For this review, take the finished solid that the model builds, in its own axes (mm). Coordinates: 2 decimals unless noted, no trailing zeros. Write each loop counter-clockwise with the first axis right and the second up, starting at its lowest first coordinate (ties: lowest second). Pieces come first, ordered by that corner, then holes. Notation, with made-up numbers: M 78.25,76 L 102.25,76 A16 cw 102.25,94 Z; hole C 17,-28.5 d10. An arc over 180 degrees is marked long. Return JSON: item names as keys, results as strings.
```python
from build123d import *

# Parameters (mm, degrees)
SKETCH1_W            = 158
SKETCH1_H            = 93
BOSS_EXTRUDE1_DEPTH  = 1.143
FILLET1_R            = 25
M4_CLEARANCE_HOLE1_D = 4.5
CHAMFER2_SIZE        = 2
CUT_EXTRUDE1_REACH   = 93.698
FILLET2_R            = 2


with BuildPart() as part:
    # Sketch1 → Boss-Extrude1 (new, symmetric)
    with BuildSketch(Plane.XY):
        Rectangle(SKETCH1_W, SKETCH1_H)
    extrude(amount=BOSS_EXTRUDE1_DEPTH, both=True)

    # Fillet1
    fillet1_edges = [part.edges().sort_by_distance(p)[0] for p in [
        (-79, 46.5, 0),
        (79, 46.5, 0),
        (79, -46.5, 0),
        (-79, -46.5, 0),
    ]]
    fillet(fillet1_edges, radius=FILLET1_R)

    # M4 Clearance Hole1 (through all)
    with Locations(Plane.XY.offset(1.143)):
        with Locations((72.5, 12.5), (0, 40), (0, -40), (-36.25, -40), (-36.25, 40), (36.25, 40), (36.25, -40), (-64.814123615, 35.759516477), (-64.814123615, -35.759516477), (64.814123615, -35.759516477), (64.814123615, 35.759516477), (-72.5, 12.5), (-72.5, -12.5), (72.5, -12.5)):
            Hole(M4_CLEARANCE_HOLE1_D / 2)

    # Chamfer2
    chamfer2_edges = [part.edges().sort_by_distance(p)[0] for p in [
        (-79, 0, 1.143),
        (0, 46.5, 1.143),
        (0, -46.5, 1.143),
        (79, 0, 1.143),
        (71.67766953, 39.17766953, 1.143),
        (-71.67766953, -39.17766953, 1.143),
        (71.67766953, -39.17766953, 1.143),
        (-71.67766953, 39.17766953, 1.143),
    ]]
    chamfer(chamfer2_edges, length=CHAMFER2_SIZE)

    # Sketch7 → Cut-Extrude1 (cut, up to next)
    with BuildSketch(Plane.XY.offset(1.143), mode=Mode.PRIVATE) as cut_extrude1_sk1:
        with BuildLine():
            Line((-33, 19.211525688), (-33, 8.788474312))
            ThreePointArc((-33, 8.788474312), (-52.4, 14), (-33, 19.211525688))
        make_face()
    cut_extrude1_tool1 = extrude(cut_extrude1_sk1.sketch, amount=-CUT_EXTRUDE1_REACH, mode=Mode.PRIVATE) & part.part
    # Sketch7 → Cut-Extrude1 (cut, up to next)
    with BuildSketch(Plane.XY.offset(1.143), mode=Mode.PRIVATE) as cut_extrude1_sk2:
        with BuildLine():
            Line((-29.633180425, -5.65), (-22.366819575, -5.65))
            ThreePointArc((-22.366819575, -5.65), (-26, -22.15), (-29.633180425, -5.65))
        make_face()
    cut_extrude1_tool2 = extrude(cut_extrude1_sk2.sketch, amount=-CUT_EXTRUDE1_REACH, mode=Mode.PRIVATE) & part.part
    # Sketch7 → Cut-Extrude1 (cut, up to next)
    with BuildSketch(Plane.XY.offset(1.143), mode=Mode.PRIVATE) as cut_extrude1_sk3:
        with BuildLine():
            Line((-1, 19.211525688), (-1, 8.788474312))
            ThreePointArc((-1, 8.788474312), (-20.4, 14), (-1, 19.211525688))
        make_face()
    cut_extrude1_tool3 = extrude(cut_extrude1_sk3.sketch, amount=-CUT_EXTRUDE1_REACH, mode=Mode.PRIVATE) & part.part
    # Sketch7 → Cut-Extrude1 (cut, up to next)
    with BuildSketch(Plane.XY.offset(1.143), mode=Mode.PRIVATE) as cut_extrude1_sk4:
        with BuildLine():
            Line((31.197, 15.790698663), (31.197, 4.209301337))
            ThreePointArc((31.197, 4.209301337), (42.5, -2.7), (53.803, 4.209301337))
            Line((53.803, 4.209301337), (53.803, 15.790698663))
            ThreePointArc((53.803, 15.790698663), (42.5, 22.7), (31.197, 15.790698663))
        make_face()
    cut_extrude1_tool4 = extrude(cut_extrude1_sk4.sketch, amount=-CUT_EXTRUDE1_REACH, mode=Mode.PRIVATE) & part.part
    # Sketch7 → Cut-Extrude1 (cut, up to next)
    with BuildSketch(Plane.XY.offset(1.143), mode=Mode.PRIVATE) as cut_extrude1_sk5:
        with BuildLine():
            Line((9.49200639, -2.65), (19.50799361, -2.65))
            ThreePointArc((19.50799361, -2.65), (14.5, -23.55), (9.49200639, -2.65))
        make_face()
    cut_extrude1_tool5 = extrude(cut_extrude1_sk5.sketch, amount=-CUT_EXTRUDE1_REACH, mode=Mode.PRIVATE) & part.part
    add(cut_extrude1_tool1.solids().sort_by_distance((-42.286012, 14, 1.143))[0], mode=Mode.SUBTRACT)
    add(cut_extrude1_tool2.solids().sort_by_distance((-26, -13.638318, 1.143))[0], mode=Mode.SUBTRACT)
    add(cut_extrude1_tool3.solids().sort_by_distance((-10.286012, 14, 1.143))[0], mode=Mode.SUBTRACT)
    add(cut_extrude1_tool4.solids().sort_by_distance((42.5, 10, 1.143))[0], mode=Mode.SUBTRACT)
    add(cut_extrude1_tool5.solids().sort_by_distance((14.5, -12.722997, 1.143))[0], mode=Mode.SUBTRACT)

    # Fillet2
    fillet2_edges = [part.edges().sort_by_distance(p)[0] for p in [
        (31.197, 15.790698663, 0),
        (53.803, 15.790698663, 0),
        (53.803, 4.209301337, 0),
        (31.197, 4.209301337, 0),
        (19.50799361, -2.65, 0),
        (9.49200639, -2.65, 0),
        (-1, 8.788474312, 0),
        (-1, 19.211525688, 0),
        (-33, 8.788474312, 0),
        (-33, 19.211525688, 0),
        (-22.366819575, -5.65, 0),
        (-29.633180425, -5.65, 0),
    ]]
    fillet(fillet2_edges, radius=FILLET2_R)


solid = part.part
```
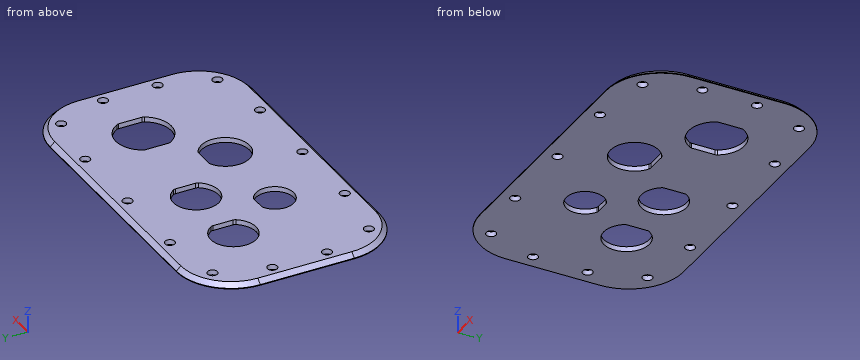
1. Clearance check with flat-ended pins moving along their axes: pin 1 Ø7 at (x, y) = (-64.81, 35.76) entering from -Z; pin 2 Ø4 at (x, y) = (72.5, -12.5) entering from -Z; pin 3 Ø1.1 at (y, z) = (10.5, 0.5) entering from -X. State where each tip first meets the part, or that it passes through.
Checks:
{"pin 1": "z = -1.14", "pin 2": "through", "pin 3": "x = -78.19"}
2. We need section D-D (z = 0.4). Give the number of separate pieces and of enclosed holes in the cut face, plus the area to 3 significant figures.
Checks:
{"separate pieces": "1", "enclosed holes": "19", "area": "11,600 mm2"}
3. Wall thickness on L1, parallel to X at y = -37, z = 0.2; L2, parallel to X at y = -7.5, z = -0.4; L3, parallel to X at y = 14, z = -0.6: over which ranges is each line inside the solid? List them lowest first. Write a range as from..to.
Checks:
{"L1": "-72.25..-66.69, -62.94..62.94, 66.69..72.25", "L2": "-78.54..-32.23, -19.77..4.65, 24.35..78.54", "L3": "-78.74..-74.18, -70.82..-52.4, -33..-20.4, -1..31.2, 53.8..70.82, 74.18..78.74"}
4. We need section C-C (x = 50). State the section outline as (y, z) points.
Checks:
{"outline": "M -46.5,-1.14 L -0.25,-1.14 L -0.25,1.14 L -44.5,1.14 L -46.5,-0.86 Z; M 20.25,-1.14 L 46.5,-1.14 L 46.5,-0.86 L 44.5,1.14 L 20.25,1.14 Z"}
5. We need section B-B (y = -12.5). State the section outline as (x, z) points.
Checks:
{"outline": "M -79,-1.14 L -74.75,-1.14 L -74.75,1.14 L -77,1.14 L -79,-0.86 Z; M -70.25,-1.14 L -34.59,-1.14 L -34.59,1.14 L -70.25,1.14 Z; M -17.41,-1.14 L 3.45,-1.14 L 3.45,1.14 L -17.41,1.14 Z; M 25.55,-1.14 L 70.25,-1.14 L 70.25,1.14 L 25.55,1.14 Z; M 74.75,-1.14 L 79,-1.14 L 79,-0.86 L 77,1.14 L 74.75,1.14 Z"}
6. We need section A-A (x = 14.5). State the section outline as (y, z) points.
Checks:
{"outline": "M -46.5,-1.14 L -23.55,-1.14 L -23.55,1.14 L -44.5,1.14 L -46.5,-0.86 Z; M -2.65,-1.14 L 46.5,-1.14 L 46.5,-0.86 L 44.5,1.14 L -2.65,1.14 Z"}
